Build history of the part. All positions in model axes, mm. Face numbers are marked on the shaded views. A direction names the side the tool comes from. Round coordinates to 2 decimals unless told otherwise and drop trailing zeros. Order: outer loops, then holes, each group sorted by start corner. A loop starts at its lowest first (then second) coordinate and runs counter-clockwise, first axis right, second up. Notation, with made-up numbers: (51.5, 59.5) -> (89.5, 59.5) arc R17 cw to (89.5, 86.5) -> close; hole circle Ø11 at (-30, 38). An arc over 180 degrees is marked (long way). Use a Markdown table: item, result. Add a question column.
Item 1: Slice it at A-A, the plane z = 4.8. Give the cut face in (x, y), plus the area to 3 significant figures.
Item 2: Slice it at B-B, the plane x = -22. Give the cut face in (y, z).
Item 3: Pin check, flat tip, straight feed: pin 1 (0.6 mm diameter, centred on y = 1, z = 2, fed in from -X). Stop position of the tip, or through.
Item 4: 3-axis set-ups, long thin cutter, end or side, ignore diameter. For the marked faces 1 and 2: which of +Z, -Z, +X, -X, +Y, -Y reach the whole face in a straight line?
Item 5: Two-plate mould, pull along X, no slides. Class the marked faces 3, 4 and 5: released by +X, released by -X, zero draft, split by the parting line, or undercut.
Item 6: Probe L1, parallel to Y at x = 8, z = 3.9; L2, parallel to X at y = -10.5, z = 2.85; L3, parallel to X at y = -11.75, z = 5.15. List the from-to ranges inside material, lowest first.
Item 7: Slice it at C-C, the plane x = -30. Give the cut face in (y, z), plus the area to 3 significant figures.
Item 8: Slice it at D-D, the plane y = -2.5. Give the cut face in (x, z).
Autodesk Inventor part; units mm, degrees
ref_plane "YZ Plane" through (0, 0, 0) normal (1, 0, 0) x (0, 1, 0)
ref_plane "XZ Plane" through (0, 0, 0) normal (0, 1, 0) x (-1, 0, 0)
ref_plane "XY Plane" through (0, 0, 0) normal (0, 0, 1) x (1, 0, 0)
sketch "Sketch1" plane through (0, 0, 0) normal (0, 0, 1) x (1, 0, 0)
  line L0 (8, 8.75) -> (8, 11) construction
  line L1 (8, 11) -> (5.7378, 11) construction
  line L2 (5.7378, 11) -> (5.7378, 8) construction
  line L3 (5.7378, 8) -> (3.2622, 8) construction
  line L4 (3.2622, 8) -> (3.2622, 11) construction
  line L5 (3.2622, 11) -> (-17.2622, 11) construction
  line L6 (-17.2622, 11) -> (-17.2622, 8) construction
  line L7 (-17.2622, 8) -> (-19.7378, 8) construction
  line L8 (-19.7378, 8) -> (-19.7378, 11) construction
  line L9 (-19.7378, 11) -> (-22.75, 11) construction
  line L10 (-25.75, 14) -> (-22.75, 11) construction
  line L11 (-25.75, 14) -> (-25.75, 0) construction
  arc A0 (-25.75, 0) -> (-22, -3.75) centre (-22, 0) ccw construction
  line L12 (-22, -3.75) -> (-20.3954, -3.75) construction
  arc A1 (-16.2094, -6.0156) -> (-20.3954, -3.75) centre (-20.3954, -8.75) ccw construction
  arc A2 (-16.2094, -6.0156) -> (2.2094, -6.0156) centre (-7, 0) ccw construction
  arc A3 (6.3954, -3.75) -> (2.2094, -6.0156) centre (6.3954, -8.75) ccw construction
  line L13 (6.3954, -3.75) -> (8, -3.75) construction
  arc A4 (8, -3.75) -> (11.75, 0) centre (8, 0) ccw construction
  line L14 (11.75, 0) -> (11.75, 7) construction
  line L15 (11.75, 7) -> (9.75, 7) construction
  line L16 (9.75, 7) -> (8, 8.75) construction
  circle A5 centre (-7, 0) radius 8.2 construction
  circle A6 centre (8, 0) radius 1.75 construction
  circle A7 centre (-22, 0) radius 1.75 construction
  circle A8 centre (-22, 0) radius 1.7
  circle A9 centre (8, 0) radius 1.7
  line L17 (-33, 0) -> (-33, -12)
  line L18 (-29, -16) -> (8, -16)
  line L19 (12, -12) -> (12, 0)
  line L20 (15, 5) -> (-29, 5) construction
  circle A10 centre (-29, 0) radius 1.7
  circle A11 centre (-29, -12) radius 1.7
  circle A12 centre (8, -12) radius 1.7
  arc A13 (-29, 4) -> (-33, 0) centre (-29, 0) ccw
  arc A14 (12, 0) -> (8, 4) centre (8, 0) ccw
  arc A15 (8, -16) -> (12, -12) centre (8, -12) ccw
  arc A16 (-33, -12) -> (-29, -16) centre (-29, -12) ccw
  line L21 (-13.2, 0) -> (-13.2, 2)
  line L22 (-0.8, 2) -> (-0.8, 0)
  line L23 (8, 4) -> (1.2, 4)
  line L24 (-15.2, 4) -> (-29, 4)
  arc A17 (-13.2, 0) -> (-0.8, 0) centre (-7, 0) ccw
  arc A18 (1.2, 4) -> (-0.8, 2) centre (1.2, 2) ccw
  arc A19 (-13.2, 2) -> (-15.2, 4) centre (-15.2, 2) ccw
  line L25 (-7, 0) -> (-7, -14.8436)
  circle A20 centre (-29, 0) radius 3 construction
  point P0 (0, 0)
  point P1 (-7, -3)
  dimension "d1" = 3.4
  dimension "d2" = 3.4
  dimension "d7" = 3.4
  dimension "d8" = 3.4
  dimension "d10" = 3.4
  dimension "d11" = 4
  dimension "d13" = 2
  dimension "d16" = 6.2
  dimension "d20" = 37
  dimension "d21" = 12
  dimension "d23" = 4
  dimension "d24" = 6
extrude "Extrusion1" add sketch "Sketch1" along normal blind 6
properties part number "Extruder_clamp"
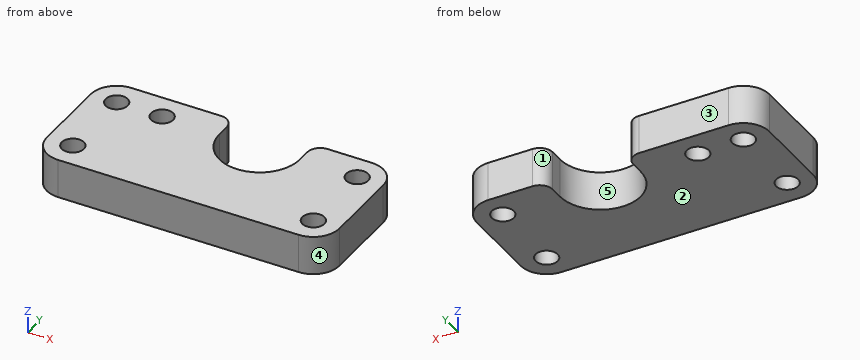
Check sheet entries:
| question | item | result |
|---|---|---|
| 1 | outline | (-33, -12) arc R4 ccw to (-29, -16) -> (8, -16) arc R4 ccw to (12, -12) -> (12, 0) arc R4 ccw to (8, 4) -> (1.2, 4) arc R2 ccw to (-0.8, 2) -> (-0.8, 0) arc R6.2 cw to (-13.2, 0) -> (-13.2, 2) arc R2 ccw to (-15.2, 4) -> (-29, 4) arc R4 ccw to (-33, 0) -> close; hole circle Ø3.4 at (-29, -12); hole circle Ø3.4 at (-29, 0); hole circle Ø3.4 at (-22, 0); hole circle Ø3.4 at (8, -12); hole circle Ø3.4 at (8, 0) |
| 1 | area | 729 mm2 |
| 2 | outline | (-16, 0) -> (-1.7, 0) -> (-1.7, 6) -> (-16, 6) -> close; (1.7, 0) -> (4, 0) -> (4, 6) -> (1.7, 6) -> close |
| 3 | pin 1 | x = -32.94 |
| 4 | face 1 | +Z, -Z, +Y |
| 4 | face 2 | -Z, +X, -X, +Y, -Y |
| 5 | face 3 | zero draft |
| 5 | face 4 | released by +X |
| 5 | face 5 | undercut |
| 6 | L1 | -16 to -13.7, -10.3 to -1.7, 1.7 to 4 |
| 6 | L2 | -33 to -29.8, -28.2 to 7.2, 8.8 to 12 |
| 6 | L3 | -33 to -30.68, -27.32 to 6.32, 9.68 to 12 |
| 7 | outline | (-15.87, 0) -> (-13.37, 0) -> (-13.37, 6) -> (-15.87, 6) -> close; (-10.63, 0) -> (-1.37, 0) -> (-1.37, 6) -> (-10.63, 6) -> close; (1.37, 0) -> (3.87, 0) -> (3.87, 6) -> (1.37, 6) -> close |
| 7 | area | 85.5 mm2 |
| 8 | outline | (-33, 0) -> (-12.67, 0) -> (-12.67, 6) -> (-33, 6) -> close; (-1.33, 0) -> (12, 0) -> (12, 6) -> (-1.33, 6) -> close |
